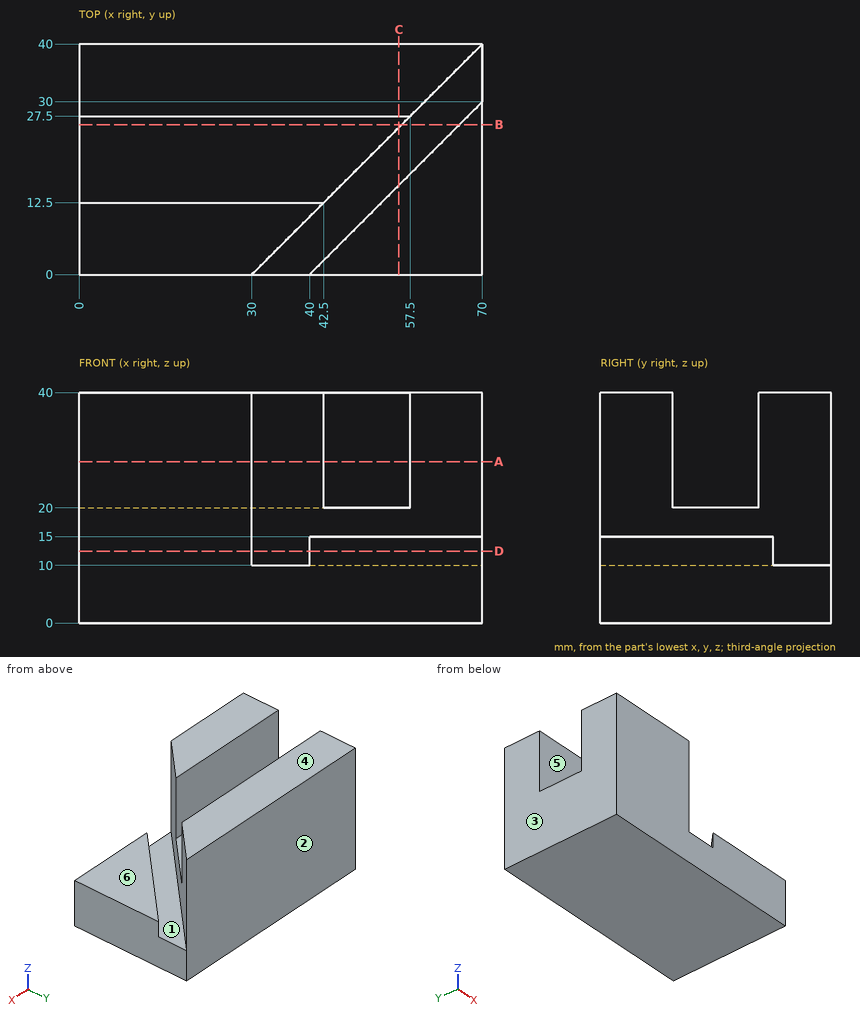
Source: three-view drawing plus pictorial views. Frame: mm from the lowest corner of the part. A direction names the side the tool comes from. Round coordinates to 2 decimals unless told otherwise and drop trailing zeros. Loops run counter-clockwise (first coordinate to the right, second up) from the corner with the lowest first, then second, coordinate; pieces in that order, holes last.
1. Section query B-B on y = 26. Output: boundary loops of the cut face in (x, z).
2. Section query C-C on x = 55.5. Output: boundary loops of the cut face in (y, z), and give its area (4 significant figures).
3. Ray query, L1, parallel to Y at x = 29.5, z = 24.5; L2, parallel to Y at x = 49, z = 25.5; L3, parallel to Y at x = 38, z = 33. Return the intervals inside material, ascending.
4. Contact query for flat-ended pins moving along their axis: pin 1 (10 mm diameter, centred on x = 41, z = 31.5, fed in from -Y); pin 2 (9 mm diameter, centred on x = 48.5, y = 20, fed in from +Z). Output: stop coordinate, or through.
5. Section query A-A on z = 28. Output: boundary loops of the cut face in (x, y), and give its area (3 significant figures).
6. Mould query, pull axis Y, two halves, no side actions, for the marked faces 1, 2 and 3. Classes: released by +Y, released by -Y, zero draft, split by the parting line, or undercut.
7. Access query for the marked faces 4, 5 and 6. Directions: +Z, -Z, +X, -X, +Y, -Y. A direction counts if a zero-diameter tool reaches every point of the face in a straight line with its end or side. Return the directions, or none.
8. Section query D-D on z = 12.5. Output: boundary loops of the cut face in (x, y).
Answers below:
1. outline: (0, 0) - (70, 0) - (70, 15) - (66, 15) - (66, 10) - (56, 10) - (56, 20) - (0, 20) - close
2. outline: (0, 0) - (40, 0) - (40, 40) - (27.5, 40) - (27.5, 20) - (25.5, 20) - (25.5, 10) - (15.5, 10) - (15.5, 15) - (0, 15) - close
2. area: 872.5 mm2
3. L1: y = 0 to 12.5, 27.5 to 40
3. L2: y = 27.5 to 40
3. L3: y = 8 to 12.5, 27.5 to 40
4. pin 1: stops at y = 6
4. pin 2: stops at z = 20
5. outline: (0, 0) - (30, 0) - (42.5, 12.5) - (0, 12.5) - close; (0, 27.5) - (57.5, 27.5) - (70, 40) - (0, 40) - close
5. area: 1,250 mm2
6. face 1: undercut
6. face 2: released by +Y
6. face 3: zero draft
7. face 4: +Z, +X, -X, +Y, -Y
7. face 5: +Z, +X, -X
7. face 6: +Z, +X, -Y
8. outline: (0, 0) - (30, 0) - (70, 40) - (0, 40) - close; (40, 0) - (70, 0) - (70, 30) - close
